from build123d import *

# Parameters (mm, degrees)
SKETCH1_W           = 10
SKETCH1_H           = 20
BOSS_EXTRUDE1_DEPTH = 7.5
SKETCH2_R           = 2.5
BOSS_EXTRUDE2_DEPTH = 1
SKETCH3_R           = 2
CUT_EXTRUDE1_DEPTH  = 1
SKETCH4_R           = 0.5
BOSS_EXTRUDE3_DEPTH = 1
SKETCH22_W          = 1.536676655
SKETCH22_H          = 12.700180583
BOSS_EXTRUDE4_DEPTH = 3.5
SKETCH25_W          = 2.5
SKETCH25_H          = 10.700180583
CUT_EXTRUDE4_DEPTH  = 5
FILLET1_R           = 2
FILLET2_R           = 2
FILLET3_R           = 2
FILLET4_R           = 2
SKETCH26_W          = 4
SKETCH26_H          = 4
BOSS_EXTRUDE5_DEPTH = 2


with BuildPart() as part:
    # Sketch1 → Boss-Extrude1 (new body)
    with BuildSketch(Plane.XY):
        with Locations((5, 10)):
            Rectangle(SKETCH1_W, SKETCH1_H)
    extrude(amount=BOSS_EXTRUDE1_DEPTH)

    # Sketch2 → Boss-Extrude2 (add)
    with BuildSketch(Plane.XY.offset(7.5)):
        with Locations(Location((4.806301262, 15.681829646, 0), (0, 0, 180))):
            Circle(SKETCH2_R)
    boss_extrude2 = extrude(amount=BOSS_EXTRUDE2_DEPTH)

    # Sketch3 → Cut-Extrude1 (cut)
    with BuildSketch(Plane.XY.offset(8.5)):
        with Locations((4.806301262, 15.681829646)):
            Circle(SKETCH3_R)
    cut_extrude1 = extrude(amount=-CUT_EXTRUDE1_DEPTH, mode=Mode.SUBTRACT)

    # Mirror1: Boss-Extrude2, Cut-Extrude1 across plane
    add(boss_extrude2.mirror(Plane.ZX.offset(10)))
    add(cut_extrude1.mirror(Plane.ZX.offset(10)), mode=Mode.SUBTRACT)

    # Sketch4 → Boss-Extrude3 (add)
    with BuildSketch(Plane(origin=(0, 20, 0), x_dir=(1, 0, 0), z_dir=(0, 1, 0))):
        with Locations(Location((4.806301262, -3.75, 0), (0, 0, 90))):
            Circle(SKETCH4_R)
    extrude(amount=BOSS_EXTRUDE3_DEPTH)

    # Loft1: read off the stored shape, not the designer's step
    # Loft1: loft between two sections, ruled curve by curve
    loft1_from = [
        Edge.make_bspline([(5.062712373, 21, 4.179247414), (5.921207201, 21, 3.666425193), (5.408384979, 21, 2.807930365), (4.549890151, 21, 3.320752586), (3.691395324, 21, 3.833574807), (4.204217545, 21, 4.692069635), (5.062712373, 21, 4.179247414)], [0, 0, 0, 0, 0.5, 0.5, 0.5, 1, 1, 1, 1], 3, [1, 0.333333333, 0.333333333, 1, 0.333333333, 0.333333333, 1]),
    ]
    loft1_to = [
        Edge.make_bspline([(4.701236965, 27.5, 4.1359553), (5.473147564, 27.5, 4.346083894), (5.683276159, 27.5, 3.574173295), (4.911365559, 27.5, 3.3640447), (4.13945496, 27.5, 3.153916106), (3.929326365, 27.5, 3.925826705), (4.701236965, 27.5, 4.1359553)], [0, 0, 0, 0, 0.5, 0.5, 0.5, 1, 1, 1, 1], 3, [1, 0.333333333, 0.333333333, 1, 0.333333333, 0.333333333, 1]),
    ]
    loft1 = Solid(Shell([*[Face.make_surface_from_curves(loft1_from[k], loft1_to[k]) for k in range(1)], Face(Wire(loft1_from)), Face(Wire(loft1_to))]))
    add(loft1)

    # Sketch20 → Revolve1 (revolve)
    with BuildSketch(Plane.XY.offset(3.75), mode=Mode.PRIVATE) as revolve1_sk:
        with BuildLine():
            Line((4.806301262, 28), (4.806301262, 27.5))
            Line((4.806301262, 27.5), (4.306301262, 27.5))
            ThreePointArc((4.306301262, 27.5), (4.452747871, 27.853553391), (4.806301262, 28))
        make_face()
    revolve(revolve1_sk.sketch.rotate(Axis((4.806301262, 28, 3.75), (0, -1, 0)), 180), axis=Axis((4.806301262, 28, 3.75), (0, -1, 0)))

    # Sketch22 → Boss-Extrude4 (add)
    with BuildSketch(Plane(origin=(10, 0, 0), x_dir=(0, 0, -1), z_dir=(1, 0, 0))):
        with Locations((-3.61725079, 10.452084784)):
            Rectangle(SKETCH22_W, SKETCH22_H)
    extrude(amount=BOSS_EXTRUDE4_DEPTH)

    # Sketch25 → Cut-Extrude4 (cut)
    with BuildSketch(Plane.XY.offset(4.385589117)):
        with Locations((11.25, 10.452084784)):
            Rectangle(SKETCH25_W, SKETCH25_H)
    extrude(amount=-CUT_EXTRUDE4_DEPTH, mode=Mode.SUBTRACT)

    # Fillet1
    fillet1_edges = [part.edges().sort_by_distance(p)[0] for p in [
        (13.5, 16.802175075, 3.617250789),
    ]]
    fillet(fillet1_edges, radius=FILLET1_R)

    # Fillet2
    fillet2_edges = [part.edges().sort_by_distance(p)[0] for p in [
        (12.5, 15.802175075, 3.617250789),
    ]]
    fillet(fillet2_edges, radius=FILLET2_R)

    # Fillet3
    fillet3_edges = [part.edges().sort_by_distance(p)[0] for p in [
        (13.5, 4.101994492, 3.617250789),
    ]]
    fillet(fillet3_edges, radius=FILLET3_R)

    # Fillet4
    fillet4_edges = [part.edges().sort_by_distance(p)[0] for p in [
        (12.5, 5.101994492, 3.617250789),
    ]]
    fillet(fillet4_edges, radius=FILLET4_R)

    # Sketch26 → Boss-Extrude5 (add)
    with BuildSketch(Plane(origin=(0, 0, 0), x_dir=(-1, 0, 0), z_dir=(0, 0, -1))):
        with Locations((-4.478821767, 10.486042594)):
            Rectangle(SKETCH26_W, SKETCH26_H)
    extrude(amount=BOSS_EXTRUDE5_DEPTH)


solid = part.part
Build history of the part. All positions in model axes, mm. A direction names the side the tool comes from. Coordinates: 2 decimals unless noted, no trailing zeros. Order: outer loops, then holes, each group sorted by start corner. A loop starts at its lowest first (then second) coordinate and runs counter-clockwise, first axis right, second up. Notation, with made-up numbers: (46.25, 89) - (103.25, 89) arc R13 ccw to (103.25, 100) - close; hole circle Ø4 at (-27, -17). An arc over 180 degrees is marked (long way). Write each question's results on one line, items separated by ' | '. Start each with the question number.
Item 1: Band-saw the part on D-D on y = 19.5. Write the cut outline in (x, z).
Item 2: Band-saw the part on A-A on y = 12. Write the cut outline in (x, z).
Item 3: Tool access for faces 1 (the face through (5, 8.486, -1)), 2 (the face through (4.37, 13.73, 8.01)), 3 (the face through (6.479, 10, -1)), 4 (the face through (11.9, 15.23, 3.61)): list every direction of +Z, -Z, +X, -X, +Y, -Y with a clear straight run to the whole face (end or side of a thin tool).
Item 4: Mould opens along Y. For faces 5 (the face through (12.5, 10, 4)), 6 (the face through (13.5, 11, 4)), 7 (the face through (5, 0, 4)) say: released by +Y, released by -Y, zero draft, split by the parting line, or undercut.
Item 5: Band-saw the part on B-B on x = 3.5. Write the cut outline in (y, z), and give its area (3 significant figures).
Item 6: Flat gauge pins, fed straight in: pin 1 (5 mm diameter, centred on x = 4.81, y = 4.32, fed in from -Z); pin 2 (1 mm diameter, centred on x = 11.5, y = 13, fed in from -Z); pin 3 (1 mm diameter, centred on x = 7, z = 4, fed in from -Y); pin 4 (0.6 mm diameter, centred on x = 10, z = 3.5, fed in from +Y). Where does each tip first touch, or does it go through?
Item 7: Band-saw the part on C-C on z = -1. Write the cut outline in (x, y).
Item 8: Wall check: probe 1 along X at (y, z) = (3.5, 2.25); probe 2 along Y at (x, z) = (4, 5.75); probe 3 along Z at (x, y) = (6.75, 10). Give the ranges that are in metal, low to high. Write a range as [from, to].
Numbers:
1) outline: (0, 0) - (10, 0) - (10, 7.5) - (0, 7.5) - close
2) outline: (0, 0) - (2.48, 0) - (2.48, -2) - (6.48, -2) - (6.48, 0) - (10, 0) - (10, 7.5) - (0, 7.5) - close; (12.5, 2.85) - (13.5, 2.85) - (13.5, 4.39) - (12.5, 4.39) - close
3) face 1: -Z, +X, -X, -Y | face 2: +Z | face 3: -Z, +X, +Y, -Y | face 4: +Z, -Z
4) face 5: undercut | face 6: zero draft | face 7: released by -Y
5) outline: (0, 0) - (8.49, 0) - (8.49, -2) - (12.49, -2) - (12.49, 0) - (20, 0) - (20, 7.5) - (17.81, 7.5) - (17.81, 8.5) - (17.2, 8.5) - (17.2, 7.5) - (14.17, 7.5) - (14.17, 8.5) - (13.55, 8.5) - (13.55, 7.5) - (6.45, 7.5) - (6.45, 8.5) - (5.83, 8.5) - (5.83, 7.5) - (2.8, 7.5) - (2.8, 8.5) - (2.19, 8.5) - (2.19, 7.5) - (0, 7.5) - close | area: 160 mm^2
6) pin 1: z = 0 | pin 2: through | pin 3: y = 0 | pin 4: y = 20
7) outline: (2.48, 8.49) - (6.48, 8.49) - (6.48, 12.49) - (2.48, 12.49) - close
8) probe 1: [0, 10] | probe 2: [0, 20] | probe 3: [0, 7.5]
